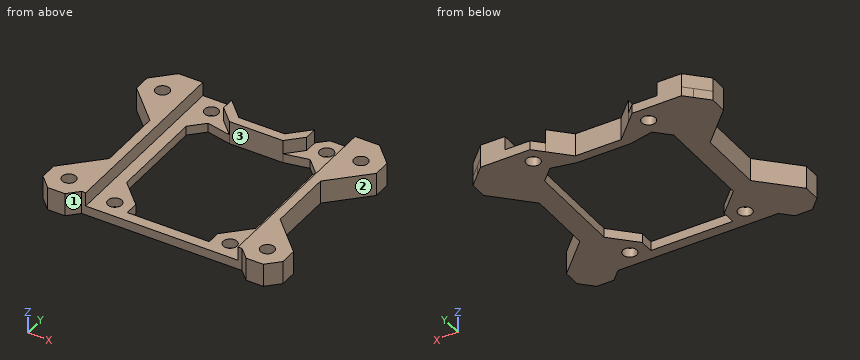
```python
from build123d import *

# Parameters (mm, degrees)
SKETCH11_R          = 1.5
BOSS_EXTRUDE4_DEPTH = 2
SKETCH12_R          = 1.5
BOSS_EXTRUDE5_DEPTH = 3


with BuildPart() as part:
    # Sketch11 → Boss-Extrude4 (new body)
    with BuildSketch(Plane.XY):
        Polygon((16.5, -2.25), (-16.5, -2.25), (-17.386038969, -2.25), (-19.636038969, -4.5), (-23.363961031, -4.5), (-26, -1.863961031), (-26, 1.863961031), (-23.363961031, 4.5), (-18.5, 9.363961031), (-18.5, 23.636038969), (-23.363961031, 28.5), (-26, 31.136038969), (-26, 34.863961031), (-23.363961031, 37.5), (-21.784271247, 39.079689783), (-13.949747468, 39.079689783), (-11.050252532, 39.079689783), (-9, 37.029437252), (-4.970562748, 33), (4.970562748, 33), (9, 37.029437252), (11.050252532, 39.079689783), (13.949747468, 39.079689783), (21.784271247, 39.079689783), (23.363961031, 37.5), (26, 34.863961031), (26, 31.136038969), (23.363961031, 28.5), (18.5, 23.636038969), (18.5, 9.363961031), (23.363961031, 4.5), (26, 1.863961031), (26, -1.863961031), (23.363961031, -4.5), (19.636038969, -4.5), (17.386038969, -2.25), align=None)
        with Locations((-12.5, 1.5)):
            Circle(SKETCH11_R, mode=Mode.SUBTRACT)
        with Locations((-12.5, 35.579689783)):
            Circle(SKETCH11_R, mode=Mode.SUBTRACT)
        with Locations(Location((12.5, 35.579689783, 0), (0, 0, 180))):
            Circle(SKETCH11_R, mode=Mode.SUBTRACT)
        with Locations(Location((12.5, 1.5, 0), (0, 0, 180))):
            Circle(SKETCH11_R, mode=Mode.SUBTRACT)
        Polygon((8.878679656, 0), (-8.878679656, 0), (-8.878679656, 3), (-11, 5.121320344), (-14, 8.121320344), (-14, 29.129942315), (-11.050252532, 32.079689783), (-5.798989873, 31), (5.798989873, 31), (11.050252532, 32.079689783), (14, 29.129942315), (14, 8.121320344), (11, 5.121320344), (8.878679656, 3), align=None, mode=Mode.SUBTRACT)
    extrude(amount=BOSS_EXTRUDE4_DEPTH)

    # Sketch12 → Boss-Extrude5 (add)
    # profile 1 of 3: a face of its own
    with BuildSketch(Plane.XY.offset(2)):
        Polygon((-23.363961031, -4.5), (-19.636038969, -4.5), (-17.386038969, -2.25), (-16.5, -2.25), (-16.5, 39.079689783), (-21.784271247, 39.079689783), (-26, 34.863961031), (-26, 31.136038969), (-18.5, 23.636038969), (-18.5, 9.363961031), (-26, 1.863961031), (-26, -1.863961031), align=None)
        with Locations((-21.5, 0)):
            Circle(SKETCH12_R, mode=Mode.SUBTRACT)
        with Locations((-21.5, 33)):
            Circle(SKETCH12_R, mode=Mode.SUBTRACT)
    # profile 2 of 3: a face of its own
    with BuildSketch(Plane.XY.offset(2)):
        Polygon((-9, 37.029437252), (-9, 34.201010127), (-5.798989873, 31), (5.798989873, 31), (9, 34.201010127), (9, 37.029437252), (4.970562748, 33), (-4.970562748, 33), align=None)
    # profile 3 of 3: a face of its own
    with BuildSketch(Plane.XY.offset(2)):
        Polygon((16.5, 39.079689783), (16.5, -2.25), (17.386038969, -2.25), (19.636038969, -4.5), (23.363961031, -4.5), (26, -1.863961031), (26, 1.863961031), (18.5, 9.363961031), (18.5, 23.636038969), (26, 31.136038969), (26, 34.863961031), (21.784271247, 39.079689783), align=None)
        with Locations((21.5, 0)):
            Circle(SKETCH12_R, mode=Mode.SUBTRACT)
        with Locations((21.5, 33)):
            Circle(SKETCH12_R, mode=Mode.SUBTRACT)
    extrude(amount=BOSS_EXTRUDE5_DEPTH)


solid = part.part
```
CAD build for the part. Positions are in the model's coordinates, mm. Face numbers are marked on the shaded views. A direction names the side the tool comes from. Coordinates: 2 decimals unless noted, no trailing zeros. Write each loop counter-clockwise with the first axis right and the second up, starting at its lowest first coordinate (ties: lowest second). Pieces come first, ordered by that corner, then holes.
(1) Cut at A-A, the plane y = 14.5. List the corners of the cut face in (x, z).
(2) Cut at B-B, the plane x = -1.5. List the corners of the cut face in (y, z), and give its area (3 significant figures).
(3) Cut at D-D, the plane x = -12.5. List the corners of the cut face in (y, z), and give its area (3 significant figures).
(4) 3-axis set-ups, long thin cutter, end or side, ignore diameter. For the marked faces 1, 2 and 3: which of +Z, -Z, +X, -X, +Y, -Y reach the whole face in a straight line?
(5) Flat gauge pins, fed straight in: pin 1 (2 mm diameter, centred on x = 13.5, y = 2, fed in from +Z); pin 2 (1 mm diameter, centred on x = -0.5, z = 1, fed in from -Y); pin 3 (10 mm diameter, centred on x = 8, y = 16.5, fed in from -Z); pin 4 (2 mm diameter, centred on y = 10, z = 1, fed in from +X). Where does each tip first touch, or does it go through?
(6) Cut at C-C, the plane z = 2.7. Count the separate pieces of the cut face and the enclosed holes in it, and give its area (3 significant figures).
(7) Drill centre lines: probe 1 along X at (y, z) = (19, 0.95); probe 2 along Y at (x, z) = (12.5, 0.95); probe 3 along Y at (x, z) = (21.5, 2.8). Where is each one in solid material? Low to high.
Geometry says:
1. outline: (-18.5, 0) - (-14, 0) - (-14, 2) - (-16.5, 2) - (-16.5, 5) - (-18.5, 5) - close; (14, 0) - (18.5, 0) - (18.5, 5) - (16.5, 5) - (16.5, 2) - (14, 2) - close
2. outline: (-2.25, 0) - (0, 0) - (0, 2) - (-2.25, 2) - close; (31, 0) - (33, 0) - (33, 5) - (31, 5) - close
2. area: 14.5 mm2
3. outline: (-2.25, 0) - (0, 0) - (0, 2) - (-2.25, 2) - close; (3, 0) - (6.62, 0) - (6.62, 2) - (3, 2) - close; (30.63, 0) - (34.08, 0) - (34.08, 2) - (30.63, 2) - close; (37.08, 0) - (39.08, 0) - (39.08, 2) - (37.08, 2) - close
3. area: 22.6 mm2
4. face 1: +Z, -Z, -Y
4. face 2: +Z, -Z, +X
4. face 3: +Z, -Z
5. pin 1: stops at z = 2
5. pin 2: stops at y = -2.25
5. pin 3: passes through
5. pin 4: stops at x = 18.86
6. separate pieces: 3
6. enclosed holes: 4
6. area: 481 mm2
7. probe 1: x = -18.5 to -14, 14 to 18.5
7. probe 2: y = -2.25 to 0, 3 to 6.62, 30.63 to 34.08, 37.08 to 39.08
7. probe 3: y = -4.5 to -1.5, 1.5 to 6.36, 26.64 to 31.5, 34.5 to 39.08
